CAD build for the part. Positions are in the model's coordinates, mm. A direction names the side the tool comes from. Give positions to 0.01 mm unless a question says otherwise; leave off trailing zeros. Loops run counter-clockwise (first coordinate to the right, second up) from the corner with the lowest first, then second, coordinate; pieces in that order, holes last.
Item 1: Probe probe 1 along Y at (x, z) = (46.25, -30); probe 2 along X at (y, z) = (12.5, -11); probe 3 along Z at (x, y) = (46.25, 0). List the from-to ranges inside material, lowest first.
Item 2: Drop flat-ended pins along their axis: P1, Ø8, axis at y = 10, z = -14, coming from the -X side; P2, Ø1, axis at x = -38, y = 30.5, coming from the +Z side; P3, Ø1, axis at y = -4.5, z = 1.5, coming from the -X side; P4, Ø4, axis at y = 28.5, z = 5.5, coming from the +X side. Give the stop position or say it passes through.
Item 3: Mould opens along Y. For faces 1 (the flat face through (-35, -1, -53)), 2 (the cylindrical face through (42.6, -0.88, -69.99)), 3 (the cylindrical face through (42.6, -2.6, -10.17)), 4 (the cylindrical face through (-14.985, 0.66, -4.93)) say: released by +Y, released by -Y, zero draft, split by the parting line, or undercut.
Item 4: Saw through at A-A on x = 0. Give the cut face in (y, z).
Item 5: Saw through at C-C on y = -10.5. Give the cut face in (x, z), plus the area to 3 significant figures.
Item 6: Saw through at B-B on z = -37.5. Give the cut face in (x, y).
Item 7: Saw through at D-D on x = -43. Give the cut face in (y, z).
Item 8: Which spindle directions (+Z, -Z, +X, -X, +Y, -Y) get a long thin tool onto all of the face, cutting with end or side? Do faces 5 (the flat face through (35, -1, -54)), 6 (the flat face through (50, 8, -50)), 7 (the flat face through (-34, 1, 0)). Say none if no direction does.
Solid Edge part; units mm, degrees
sketch "Sketch1" plane through (0, 0, 0) normal (0, 0, 1) x (1, 0, 0)
  line L0 (-50, -40) -> (50, -40)
  line L1 (50, -40) -> (50, 40)
  line L2 (50, 40) -> (-50, 40)
  line L3 (-50, 40) -> (-50, -40)
extrude "Protrusion1" add sketch "Sketch1" against normal blind 10
sketch "Sketch2" plane through (50, 0, -5) normal (1, 0, 0) x (0, 1, 0)
  line L0 (-40, -5) -> (-40, -25)
  line L1 (40, -5) -> (-40, -5)
  line L2 (40, -25) -> (40, -5)
  arc A0 (40, -25) -> (-40, -25) centre (0, -25) cw
extrude "Protrusion_2" add sketch "Sketch2" against normal blind 15
sketch "Sketch3" plane through (-50, 0, -5) normal (-1, 0, 0) x (0, -1, 0)
  line L0 (-40, -5) -> (-40, -25)
  line L1 (40, -5) -> (-40, -5)
  line L2 (40, -25) -> (40, -5)
  arc A0 (40, -25) -> (-40, -25) centre (0, -25) cw
extrude "Protrusion_3" add sketch "Sketch3" against normal blind 15
sketch "Sketch4" plane through (50, 0, -35) normal (1, 0, 0) x (0, 1, 0)
  circle A0 centre (0, 5) radius 20
extrude "ExtrudedCutout_1" cut sketch "Sketch4" against normal blind 25.6414
sketch "Sketch5" plane through (-50, 0, -35) normal (-1, 0, 0) x (0, -1, 0)
  circle A0 centre (0, 5) radius 20
extrude "ExtrudedCutout_2" cut sketch "Sketch5" against normal blind 43.9388
sketch "Sketch6" plane through (0, 0, 0) normal (0, 0, 1) x (1, 0, 0)
  circle A0 centre (0, 0) radius 15
extrude "Cutout_3" cut sketch "Sketch6" against normal blind 37.3136
sketch "Sketch7" plane through (0, 0, 0) normal (0, 0, 1) x (1, 0, 0)
  circle A0 centre (0, 0) radius 30
  circle A1 centre (0, 0) radius 25
extrude "Protrusion_4" add sketch "Sketch7" along normal blind 20
Results below:
1. probe 1: y = -40 to -20, 20 to 40
1. probe 2: x = -50 to -35, 35 to 50
1. probe 3: z = -70 to -50, -10 to 0
2. P1: stops at x = -50
2. P2: stops at z = 0
2. P3: stops at x = -29.73
2. P4: stops at x = 14.06
3. face 1: zero draft
3. face 2: split by the parting line
3. face 3: undercut
3. face 4: undercut
4. outline: (-40, -10) - (-15, -10) - (-15, 0) - (-25, 0) - (-25, 20) - (-30, 20) - (-30, 0) - (-40, 0) - close; (15, -10) - (40, -10) - (40, 0) - (30, 0) - (30, 20) - (25, 20) - (25, 0) - (15, 0) - close
5. outline: (-50, -68.6) - (-35, -68.6) - (-35, -47.02) - (-50, -47.02) - close; (-50, -12.98) - (-35, -12.98) - (-35, -10) - (-10.71, -10) - (-10.71, 0) - (-22.69, 0) - (-22.69, 20) - (-28.1, 20) - (-28.1, 0) - (-50, 0) - close; (10.71, -10) - (35, -10) - (35, -12.98) - (50, -12.98) - (50, 0) - (28.1, 0) - (28.1, 20) - (22.69, 20) - (22.69, 0) - (10.71, 0) - close; (35, -68.6) - (50, -68.6) - (50, -47.02) - (35, -47.02) - close
5. area: 1,740 mm2
6. outline: (-50, -39.29) - (-35, -39.29) - (-35, -18.54) - (-50, -18.54) - close; (-50, 18.54) - (-35, 18.54) - (-35, 39.29) - (-50, 39.29) - close; (35, -39.29) - (50, -39.29) - (50, -18.54) - (35, -18.54) - close; (35, 18.54) - (50, 18.54) - (50, 39.29) - (35, 39.29) - close
7. outline: (-40, -30) arc R40 ccw to (40, -30) - (40, 0) - (-40, 0) - close; hole circle Ø40 at (0, -30)
8. face 5: -Z, +Y, -Y
8. face 6: +Z, -Z, +X, +Y, -Y
8. face 7: +Z
